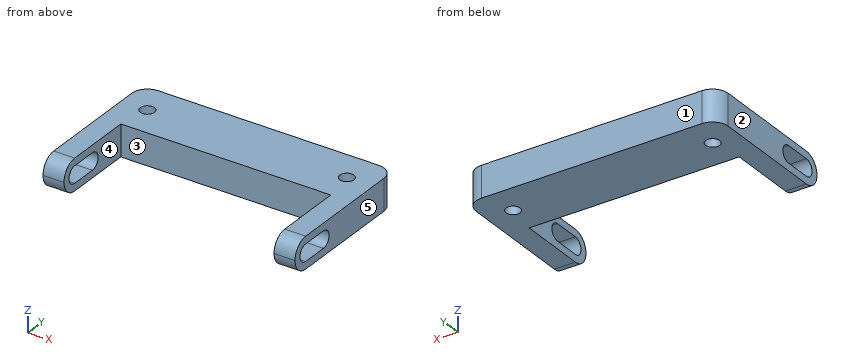
```python
from build123d import *

# Parameters (mm, degrees)
EXTRUDE_1_DEPTH     = 6
CUT_EXTRUDE_1_REACH = 55.141
FILLET_1_R          = 3
SKETCH_3_R          = 1.35
CUT_EXTRUDE_2_DEPTH = 34.105890714


with BuildPart() as part:
    # 草圖1 → 填料-伸長1 (new body)
    with BuildSketch(Plane.XY):
        Polygon((-20, -6), (20, -6), (20, -22), (24, -22), (24, -6), (24, 6), (-24, 6), (-24, -6), (-24, -22), (-20, -22), align=None)
    extrude(amount=EXTRUDE_1_DEPTH)

    # 草圖2 → 除料-伸長1 (cut, up to next)
    with BuildSketch(Plane(origin=(24, 0, 0), x_dir=(0, 0, -1), z_dir=(1, 0, 0)), mode=Mode.PRIVATE) as cut_extrude_1_sk1:
        with BuildLine():
            Line((-1.4, -14), (-1.4, -19))
            ThreePointArc((-1.4, -19), (-3, -20.6), (-4.6, -19))
            Line((-4.6, -19), (-4.6, -14))
            ThreePointArc((-4.6, -14), (-3, -12.4), (-1.4, -14))
        make_face()
    cut_extrude_1_tool1 = extrude(cut_extrude_1_sk1.sketch, amount=-CUT_EXTRUDE_1_REACH, mode=Mode.PRIVATE) & part.part
    cut_extrude_1 = cut_extrude_1_tool1.solids().sort_by_distance((24, -16.5, 3))[0]
    add(cut_extrude_1, mode=Mode.SUBTRACT)

    # 鏡射1: 除料-伸長1 across plane
    add(cut_extrude_1.mirror(Plane(origin=(0, 0, 0), x_dir=(0, 0, 1), z_dir=(1, 0, 0))), mode=Mode.SUBTRACT)

    # 圓角1
    fillet_1_edges = [part.edges().sort_by_distance(p)[0] for p in [
        (-24, 6, 3),
        (24, 6, 3),
        (-22, -22, 6),
        (-22, -22, 0),
        (22, -22, 0),
        (22, -22, 6),
    ]]
    fillet(fillet_1_edges, radius=FILLET_1_R - 0.0001)  # a hair under: the kernel refuses the full size

    # 草圖3 → 除料-伸長2 (cut, through all)
    with BuildSketch(Plane(origin=(0, 0, 0), x_dir=(-1, 0, 0), z_dir=(0, 0, -1))):
        with Locations((19, 0)):
            Circle(SKETCH_3_R)
        with Locations((-19, 0)):
            Circle(SKETCH_3_R)
    extrude(amount=-CUT_EXTRUDE_2_DEPTH, mode=Mode.SUBTRACT)


solid = part.part
```
The model under review builds one solid part; all positions refer to its coordinate system, in mm. Face numbers are marked on the shaded views. A direction names the side the tool comes from. Round coordinates to 2 decimals unless told otherwise and drop trailing zeros. Write each loop counter-clockwise with the first axis right and the second up, starting at its lowest first coordinate (ties: lowest second). Pieces come first, ordered by that corner, then holes. Notation, with made-up numbers: (-13.5, 14.25) - (1.5, 14.25) arc R8 ccw to (1.5, 26.25) - close; hole circle Ø2 at (-34, 34.5). An arc over 180 degrees is marked (long way). Use one line per item in the form item = value.
Q1. Consider section B-B (y = 0). State the section outline as (x, z) points, and give its area (3 significant figures).
Answer key:
outline = (-24, 0) - (-20.35, 0) - (-20.35, 6) - (-24, 6) - close; (-17.65, 0) - (17.65, 0) - (17.65, 6) - (-17.65, 6) - close; (20.35, 0) - (24, 0) - (24, 6) - (20.35, 6) - close
area = 256 mm2
Q2. Draft analysis for pull direction X (two halves, no side actions). For the marked faces 1, 2 and 3, state which applies: +X half, -X half, draft (parallel to the pull), parting line (faces both ways), or undercut.
Answer key:
face_1 = draft
face_2 = -X half
face_3 = undercut
Q3. Consider section C-C (y = -14.5). State the section outline as (x, z) points.
Answer key:
outline = (-24, 0) - (-20, 0) - (-20, 1.4) - (-24, 1.4) - close; (-24, 4.6) - (-20, 4.6) - (-20, 6) - (-24, 6) - close; (20, 0) - (24, 0) - (24, 1.4) - (20, 1.4) - close; (20, 4.6) - (24, 4.6) - (24, 6) - (20, 6) - close
Q4. Consider section D-D (z = 1.95). State the section outline as (x, y) points, and give its area (3 significant figures).
Answer key:
outline = (-24, -21.81) - (-20, -21.81) - (-20, -20.21) - (-24, -20.21) - close; (-24, -12.79) - (-20, -12.79) - (-20, -6) - (20, -6) - (20, -12.79) - (24, -12.79) - (24, 3) arc R3 ccw to (21, 6) - (-21, 6) arc R3 ccw to (-24, 3) - close; (20, -21.81) - (24, -21.81) - (24, -20.21) - (20, -20.21) - close; hole circle Ø2.7 at (-19, 0); hole circle Ø2.7 at (19, 0)
area = 628 mm2
Q5. Tool access review of the marked faces 4 and 5: name each direction out of +Z, -Z, +X, -X, +Y, -Y from which nothing blocks a thin tool from reaching the whole face with its end or side.
Answer key:
face_4 = +Z, -Z, -Y
face_5 = +Z, -Z, +X, +Y, -Y
Q6. Insertion check: pin 1 Ø1.8 at (x, z) = (1.5, 3.5) entering from -Y. The pin has a flat end and moves straight along its axis. Give the tip position at first contact, or say it passes through.
Answer key:
pin_1 = -6
Q7. For line 1 (X direction, y = -18, z = 5.25); line 2 (Y direction, x = 19, z = 1.85); line 3 (Z direction, x = 21, y = -14.75), list the stretches that pass through material, from the lowest coordinate up. Write a range as [from, to].
Answer key:
line_1 = [-24, -20], [20, 24]
line_2 = [-6, -1.35], [1.35, 6]
line_3 = [0, 1.4], [4.6, 6]
Q8. Consider section A-A (x = 19). State the section outline as (y, z) points.
Answer key:
outline = (-6, 0) - (-1.35, 0) - (-1.35, 6) - (-6, 6) - close; (1.35, 0) - (6, 0) - (6, 6) - (1.35, 6) - close
